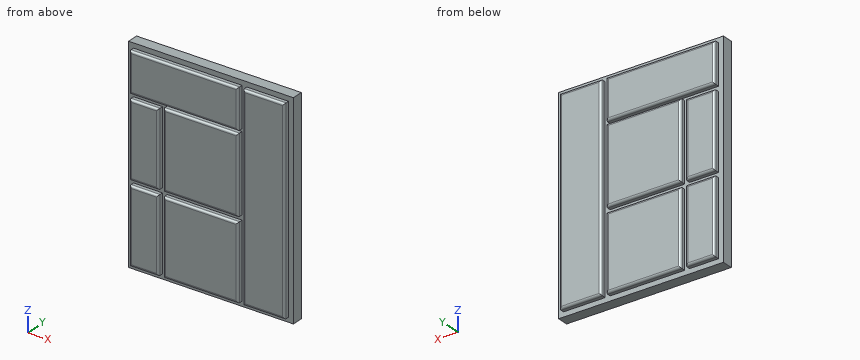
```python
from build123d import *

# Parameters (mm, degrees)
SKETCH014_W   = 75
SKETCH014_H   = 95
PAD009_DEPTH  = 2.5
SKETCH013_W   = 49.4
SKETCH013_H   = 18.2
SKETCH013_W_2 = 19
SKETCH013_H_2 = 90.6
SKETCH013_W_3 = 13.2
SKETCH013_H_3 = 34
SKETCH013_W_4 = 34
SKETCH013_H_4 = 35
PAD010_DEPTH  = 5
FILLET006_R   = 1
FILLET007_R   = 1


with BuildPart() as part:
    # Sketch014 → Pad009 (new body, symmetric)
    with BuildSketch(Plane.XZ):
        Rectangle(SKETCH014_W, SKETCH014_H)
    extrude(amount=PAD009_DEPTH, both=True)

    # Sketch013 → Pad010 (join, symmetric)
    with BuildSketch(Plane.XZ):
        with Locations((-10.6, 36.2)):
            Rectangle(SKETCH013_W, SKETCH013_H)
        with Locations((25.8, 0)):
            Rectangle(SKETCH013_W_2, SKETCH013_H_2)
        with Locations((-28.7, 7.9)):
            Rectangle(SKETCH013_W_3, SKETCH013_H_3)
        with Locations((-28.7, -28.3)):
            Rectangle(SKETCH013_W_3, SKETCH013_H_3)
        with Locations((-2.9, 8.4)):
            Rectangle(SKETCH013_W_4, SKETCH013_H_4)
        with Locations((-2.9, -28.3)):
            Rectangle(SKETCH013_W_4, SKETCH013_H_3)
    extrude(amount=PAD010_DEPTH, both=True)

    # Fillet006
    fillet006_edges = [part.edges().sort_by_distance(p)[0] for p in [
        (-10.6, -5, 45.3),
        (14.1, -5, 36.2),
        (-10.6, -5, 27.1),
        (-35.3, -5, 36.2),
        (-28.7, -5, 24.9),
        (-22.1, -5, 7.9),
        (-28.7, -5, -9.1),
        (-35.3, -5, 7.9),
        (-2.9, -5, 25.9),
        (14.1, -5, 8.4),
        (-2.9, -5, -9.1),
        (-19.9, -5, 8.4),
        (-28.7, -5, -11.3),
        (-22.1, -5, -28.3),
        (-28.7, -5, -45.3),
        (-35.3, -5, -28.3),
        (-2.9, -5, -11.3),
        (14.1, -5, -28.3),
        (-2.9, -5, -45.3),
        (-19.9, -5, -28.3),
        (25.8, -5, 45.3),
        (35.3, -5, 0),
        (25.8, -5, -45.3),
        (16.3, -5, 0),
    ]]
    fillet(fillet006_edges, radius=FILLET006_R)

    # Fillet007
    fillet007_edges = [part.edges().sort_by_distance(p)[0] for p in [
        (-10.6, 5, 45.3),
        (14.1, 5, 36.2),
        (-10.6, 5, 27.1),
        (-35.3, 5, 36.2),
        (-28.7, 5, 24.9),
        (-22.1, 5, 7.9),
        (-28.7, 5, -9.1),
        (-35.3, 5, 7.9),
        (-2.9, 5, 25.9),
        (14.1, 5, 8.4),
        (-2.9, 5, -9.1),
        (-19.9, 5, 8.4),
        (-28.7, 5, -11.3),
        (-22.1, 5, -28.3),
        (-28.7, 5, -45.3),
        (-35.3, 5, -28.3),
        (-2.9, 5, -11.3),
        (14.1, 5, -28.3),
        (-2.9, 5, -45.3),
        (-19.9, 5, -28.3),
        (25.8, 5, 45.3),
        (35.3, 5, 0),
        (25.8, 5, -45.3),
        (16.3, 5, 0),
    ]]
    fillet(fillet007_edges, radius=FILLET007_R)


solid = part.part
```
The model under review builds one solid part; all positions refer to its coordinate system, in mm. Round coordinates to 2 decimals unless told otherwise and drop trailing zeros. Write each loop counter-clockwise with the first axis right and the second up, starting at its lowest first coordinate (ties: lowest second). Pieces come first, ordered by that corner, then holes.
(1) We need section A-A on z = 30.5. Give the boundary of the cut face in (x, y), and give its area (3 significant figures).
(2) Wall thickness on L1, parallel to X at y = 3.75, z = -0.5; L2, parallel to Z at x = -29, y = 3.5; L3, parallel to Z at x = -7.5, y = -3.25: over which ranges is each line inside the solid? List them lowest first.
(3) Insertion check: pin 1 (0.8 mm diameter, centred on x = -9.5, y = 3, fed in from +Z); pin 2 (1.2 mm diameter, centred on x = -5, y = -3.5, fed in from -Z); pin 3 (1.2 mm diameter, centred on y = 3.5, z = 36.5, fed in from -X). Each pin has a flat end and moves straight along its axis. Give the tip position at first contact, or say it passes through.
(4) We need section B-B on x = 18.5. Give the boundary of the cut face in (y, z).
Findings below:
1. outline: (-37.5, -2.5) - (-35.3, -2.5) - (-35.3, -4) arc R1 ccw to (-34.3, -5) - (13.1, -5) arc R1 ccw to (14.1, -4) - (14.1, -2.5) - (16.3, -2.5) - (16.3, -4) arc R1 ccw to (17.3, -5) - (34.3, -5) arc R1 ccw to (35.3, -4) - (35.3, -2.5) - (37.5, -2.5) - (37.5, 2.5) - (35.3, 2.5) - (35.3, 4) arc R1 ccw to (34.3, 5) - (17.3, 5) arc R1 ccw to (16.3, 4) - (16.3, 2.5) - (14.1, 2.5) - (14.1, 4) arc R1 ccw to (13.1, 5) - (-34.3, 5) arc R1 ccw to (-35.3, 4) - (-35.3, 2.5) - (-37.5, 2.5) - close
1. area: 715 mm2
2. L1: x = -35.3 to -22.1, -19.9 to 14.1, 16.3 to 35.3
2. L2: z = -45.3 to -11.3, -9.1 to 24.9, 27.1 to 45.3
2. L3: z = -45.3 to -11.3, -9.1 to 25.9, 27.1 to 45.3
3. pin 1: stops at z = 45.3
3. pin 2: stops at z = -45.3
3. pin 3: stops at x = -35.3
4. outline: (-5, -44.3) arc R1 ccw to (-4, -45.3) - (-2.5, -45.3) - (-2.5, -47.5) - (2.5, -47.5) - (2.5, -45.3) - (4, -45.3) arc R1 ccw to (5, -44.3) - (5, 44.3) arc R1 ccw to (4, 45.3) - (2.5, 45.3) - (2.5, 47.5) - (-2.5, 47.5) - (-2.5, 45.3) - (-4, 45.3) arc R1 ccw to (-5, 44.3) - close
